The model under review builds one solid part; all positions refer to its coordinate system, in mm. Face numbers are marked on the shaded views. A direction names the side the tool comes from. Round coordinates to 2 decimals unless told otherwise and drop trailing zeros. Write each loop counter-clockwise with the first axis right and the second up, starting at its lowest first coordinate (ties: lowest second). Pieces come first, ordered by that corner, then holes. Notation, with made-up numbers: M 45,-5 L 64,-5 A29 cw 64,24 Z; hole C 76,-38.75 d8. An arc over 180 degrees is marked long. One line per item, written item: value. Start each with the question number.
1) For P1, Ø1, axis at x = -3, z = -26.5, coming from the +Y side, flat-tipped, find the tip position at first contact; note if it passes through.
2) Take a section at A-A, the plane x = 0. Write out the cut boundary in (y, z), and give its area (3 significant figures).
3) Tool access review of the marked faces 1 and 2: name each direction out of +Z, -Z, +X, -X, +Y, -Y from which nothing blocks a thin tool from reaching the whole face with its end or side.
4) Take a section at C-C, the plane z = -26.65. Write out the cut boundary in (x, y).
5) Take a section at D-D, the plane y = 17.5. Write out the cut boundary in (x, z), and give its area (3 significant figures).
6) Wall thickness on probe 1 along X at (y, z) = (-16, -26.75); probe 2 along Y at (x, z) = (-8, -27.6); probe 3 along X at (y, z) = (-15.5, -27.15): over which ranges is each line inside the solid? List them lowest first.
7) Take a section at B-B, the plane y = 0. Write out the cut boundary in (x, z).
from build123d import *

# Parameters (mm, degrees)
BOSS_EXTRUDE1_START     = -27
SKETCH1_R               = 21
BOSS_EXTRUDE1_DEPTH     = 1
BOSS_EXTRUDE2_START     = -27.8
SKETCH2_R               = 19
BOSS_EXTRUDE2_DEPTH     = 0.8
CUT_EXTRUDE1_DEPTH      = 41.67972468
CUT_EXTRUDE1_DEPTH_BACK = 41.67972468
SKETCH3_W               = 14
SKETCH3_H               = 60


with BuildPart() as part:
    # Sketch1 → Boss-Extrude1 (new body)
    with BuildSketch(Plane.XY.offset(BOSS_EXTRUDE1_START)):
        Circle(SKETCH1_R)
    extrude(amount=BOSS_EXTRUDE1_DEPTH)

    # Sketch2 → Boss-Extrude2 (add)
    with BuildSketch(Plane.XY.offset(BOSS_EXTRUDE2_START)):
        Circle(SKETCH2_R)
    extrude(amount=BOSS_EXTRUDE2_DEPTH)

    # Sketch3 → Cut-Extrude1 (cut, two sides: drawn at the far end of the back side and taken through both)
    with BuildSketch(Plane.XY.offset(-CUT_EXTRUDE1_DEPTH_BACK)):
        with Locations((23, 0)):
            Rectangle(SKETCH3_W, SKETCH3_H)
    extrude(amount=CUT_EXTRUDE1_DEPTH + CUT_EXTRUDE1_DEPTH_BACK, mode=Mode.SUBTRACT)


solid = part.part
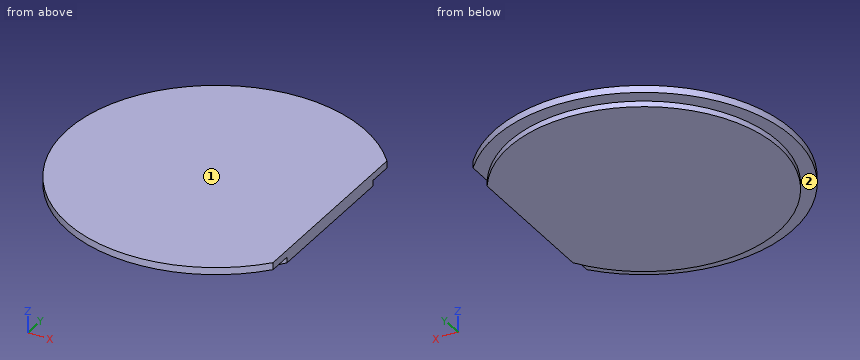
Checked values:
1. P1: stops at y = 20.85
2. outline: M -21,-27 L -19,-27 L -19,-27.8 L 19,-27.8 L 19,-27 L 21,-27 L 21,-26 L -21,-26 Z
2. area: 72.4 mm2
3. face 1: +Z, +X, -X, +Y, -Y
3. face 2: -Z
4. outline: M 16,-13.6 L 16,13.6 A21 ccw long Z
5. outline: M -11.61,-27 L -7.4,-27 L -7.4,-27.8 L 7.4,-27.8 L 7.4,-27 L 11.61,-27 L 11.61,-26 L -11.61,-26 Z
5. area: 35.1 mm2
6. probe 1: x = -13.6 to 13.6
6. probe 2: y = -17.23 to 17.23
6. probe 3: x = -10.99 to 10.99
7. outline: M -21,-27 L -19,-27 L -19,-27.8 L 16,-27.8 L 16,-26 L -21,-26 Z
